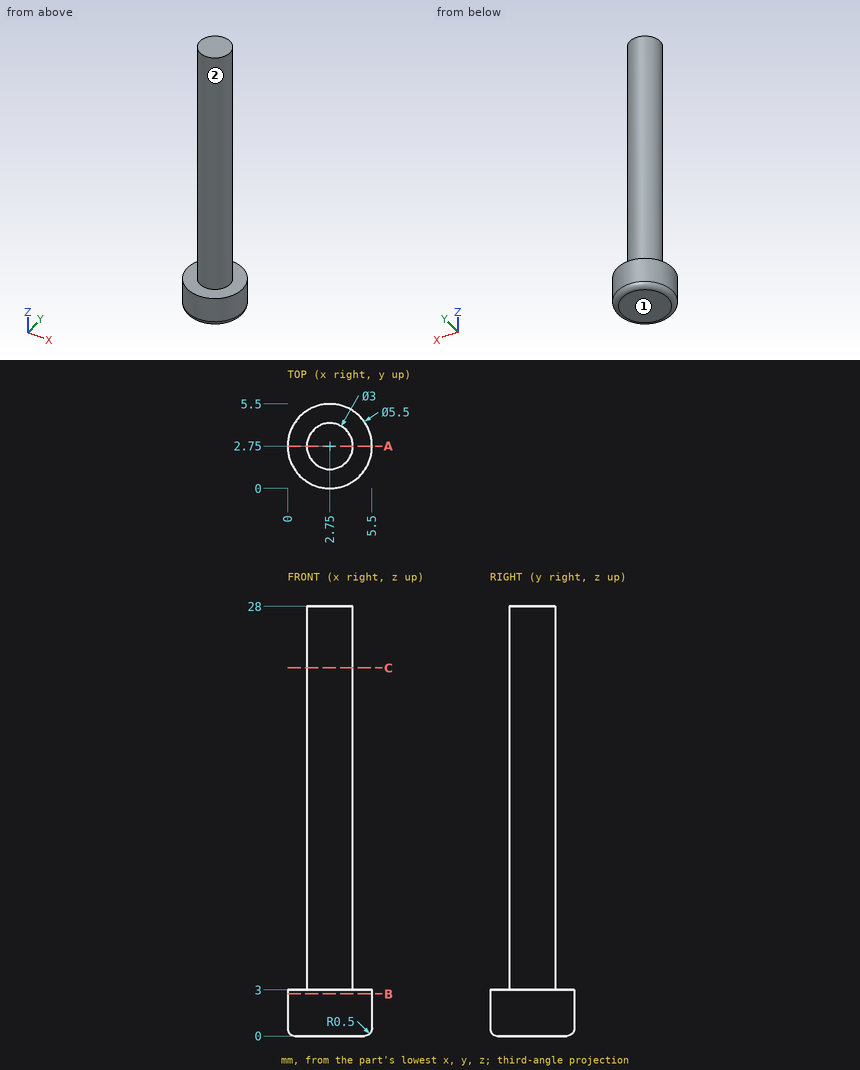
Drawing for the job (mm, zero at the part's lowest x, y, z). A direction names the side the tool comes from. Give positions to 0.01 mm unless a question says otherwise; leave off trailing zeros. Loops run counter-clockwise (first coordinate to the right, second up) from the corner with the lowest first, then second, coordinate; pieces in that order, holes last.
Item 1: Slice it at B-B (z = 2.75). Write the cut outline in (x, y).
Check values:
outline: circle Ø5.5 at (2.75, 2.75)
Item 2: Which spindle directions (+Z, -Z, +X, -X, +Y, -Y) get a long thin tool onto all of the face, cutting with end or side? Do the marked faces 1 and 2. Say none if no direction does.
Check values:
face 1: -Z, +X, -X, +Y, -Y
face 2: +Z
Item 3: Drill centre lines: line 1 along Z through (x, y) = (2.15, 4.4); line 2 along X through (y, z) = (2.7, 25); line 3 along Y through (x, z) = (3.85, 4). Where is each one in solid material? Low to high.
Check values:
line 1: z = 0 to 3
line 2: x = 1.25 to 4.25
line 3: y = 1.73 to 3.77
Item 4: Slice it at A-A (y = 2.75). Write the cut outline in (x, z), plus the area to 3 significant figures.
Check values:
outline: (0, 0.5) arc R0.5 ccw to (0.5, 0) - (5, 0) arc R0.5 ccw to (5.5, 0.5) - (5.5, 3) - (4.25, 3) - (4.25, 28) - (1.25, 28) - (1.25, 3) - (0, 3) - close
area: 91.4 mm2
Item 5: Slice it at C-C (z = 24). Write the cut outline in (x, y).
Check values:
outline: circle Ø3 at (2.75, 2.75)
Item 6: Drop flat-ended pins along their axis: P1, Ø1, axis at x = 1, z = 5, coming from the -Y side; P2, Ø3, axis at y = 1.5, z = 12, coming from the +X side; P3, Ø3, axis at x = 2.5, z = 23.5, coming from the -Y side. Give the stop position or say it passes through.
Check values:
P1: stops at y = 1.92
P2: stops at x = 4.25
P3: stops at y = 1.25
